```python
from build123d import *

# Parameters (mm, degrees)
SKETCH1_R                                       = 2.5
BOSS_EXTRUDE1_DEPTH                             = 35
CUT_EXTRUDE1_OUTLINE_W                          = 11.354248689
CUT_EXTRUDE1_OUTLINE_H                          = 14
CUT_EXTRUDE1_DEPTH                              = 10.980294351
CSK_FOR_M5_FLAT_HEAD_MACHINE_SCREW1_D           = 5.5
CSK_FOR_M5_FLAT_HEAD_MACHINE_SCREW1_DEPTH       = 13.347633298
CSK_FOR_M5_FLAT_HEAD_MACHINE_SCREW1_CSINK_D     = 10.4
CSK_FOR_M5_FLAT_HEAD_MACHINE_SCREW1_CSINK_ANGLE = 90
CSK_FOR_M5_FLAT_HEAD_MACHINE_SCREW1_TIP         = 1.652366702
SKETCH6_R                                       = 5.25
CUT_EXTRUDE2_DEPTH                              = 14
CUT_EXTRUDE3_START                              = -28
SKETCH6_2_R                                     = 5.25
CUT_EXTRUDE3_DEPTH                              = 14
CUT_EXTRUDE4_START                              = -56
SKETCH6_3_R                                     = 5.25
CUT_EXTRUDE4_DEPTH                              = 14


# Read off the part's stored shape, not the designer's step: Cut-Extrude1
with BuildPart() as part:
    # Sketch1 → Boss-Extrude1 (new, symmetric)
    with BuildSketch(Plane(origin=(0, 0, 0), x_dir=(1, 0, 0), z_dir=(0, 1, 0))):
        with BuildLine():
            Line((0, 0), (28, 0))
            Line((28, 0), (28, -1.5))
            ThreePointArc((28, -1.5), (34.920820135, -7.683011565), (25.645751311, -8))
            Line((25.645751311, -8), (2.645751311, -8))
            Line((2.645751311, -8), (0, -5))
            Line((0, -5), (0, 0))
        make_face()
        with Locations(Location((30.219676222, -5.980294351, 0), (0, 0, 270))):
            Circle(SKETCH1_R, mode=Mode.SUBTRACT)
    extrude(amount=BOSS_EXTRUDE1_DEPTH, both=True)

    # Cut-Extrude1 outline → Cut-Extrude1 (cut)
    with BuildSketch(Plane.XY):
        with Locations((31.322875655, 0)):
            Rectangle(CUT_EXTRUDE1_OUTLINE_W, CUT_EXTRUDE1_OUTLINE_H)
        with Locations((31.322875655, 28)):
            Rectangle(CUT_EXTRUDE1_OUTLINE_W, CUT_EXTRUDE1_OUTLINE_H)
        with Locations((31.322875655, -28)):
            Rectangle(CUT_EXTRUDE1_OUTLINE_W, CUT_EXTRUDE1_OUTLINE_H)
    extrude(amount=CUT_EXTRUDE1_DEPTH, mode=Mode.SUBTRACT)

    # CSK for M5 Flat Head Machine Screw1
    with Locations(Plane.XY.offset(8)):
        with Locations((12.432713767, 18), (12.432713767, -18)):
            CounterSinkHole(CSK_FOR_M5_FLAT_HEAD_MACHINE_SCREW1_D / 2, CSK_FOR_M5_FLAT_HEAD_MACHINE_SCREW1_CSINK_D / 2, depth=CSK_FOR_M5_FLAT_HEAD_MACHINE_SCREW1_DEPTH, counter_sink_angle=CSK_FOR_M5_FLAT_HEAD_MACHINE_SCREW1_CSINK_ANGLE)
            with Locations((0, 0, -(CSK_FOR_M5_FLAT_HEAD_MACHINE_SCREW1_DEPTH + CSK_FOR_M5_FLAT_HEAD_MACHINE_SCREW1_TIP / 2))):  # 118° drill point
                Cone(0, CSK_FOR_M5_FLAT_HEAD_MACHINE_SCREW1_D / 2, CSK_FOR_M5_FLAT_HEAD_MACHINE_SCREW1_TIP, mode=Mode.SUBTRACT)

    # Sketch6 → Cut-Extrude2 (cut)
    with BuildSketch(Plane(origin=(0, 35, 0), x_dir=(1, 0, 0), z_dir=(0, 1, 0))):
        with Locations((30.219676222, -5.980294351)):
            Circle(SKETCH6_R)
    extrude(amount=-CUT_EXTRUDE2_DEPTH, mode=Mode.SUBTRACT)

    # Sketch6<2> → Cut-Extrude3 (cut)
    with BuildSketch(Plane(origin=(0, 35, 0), x_dir=(1, 0, 0), z_dir=(0, 1, 0)).offset(CUT_EXTRUDE3_START)):
        with Locations((30.219676222, -5.980294351)):
            Circle(SKETCH6_2_R)
    extrude(amount=-CUT_EXTRUDE3_DEPTH, mode=Mode.SUBTRACT)

    # Sketch6<3> → Cut-Extrude4 (cut)
    with BuildSketch(Plane(origin=(0, 35, 0), x_dir=(1, 0, 0), z_dir=(0, 1, 0)).offset(CUT_EXTRUDE4_START)):
        with Locations((30.219676222, -5.980294351)):
            Circle(SKETCH6_3_R)
    extrude(amount=-CUT_EXTRUDE4_DEPTH, mode=Mode.SUBTRACT)


solid = part.part
```
The model under review builds one solid part; all positions refer to its coordinate system, in mm. A direction names the side the tool comes from. Round coordinates to 2 decimals unless told otherwise and drop trailing zeros. Order: outer loops, then holes, each group sorted by start corner. A loop starts at its lowest first (then second) coordinate and runs counter-clockwise, first axis right, second up.
Item 1: Add section A-A, the plane z = 10.25. State the section outline as (x, y) points, and give its area (3 significant figures).
Working result:
outline: (27.62, -21) - (32.82, -21) - (32.82, -7) - (27.62, -7) - close; (27.62, 7) - (32.82, 7) - (32.82, 21) - (27.62, 21) - close
area: 146 mm2
Item 2: Machinability: for faces 1 (the flat face through (1.34, 0.49, 6.52)), 2 (the flat face through (25.646, -28, 2)), 3 (the flat face through (25.646, 0, 2)), 4 (the flat face through (25.646, 28, 2)), 5 (the flat face through (13, 35, 4)), which of the approach directions +Z, -Z, +X, -X, +Y, -Y give a long, thin tool a straight path to every point of the face, cutting with its end or side? Answer none if there is none.
Working result:
face 1: +Z, -X, +Y, -Y
face 2: +Z, -Z, +X, -Y
face 3: +Z, -Z, +X
face 4: +Z, -Z, +X, +Y
face 5: +Z, -Z, +X, -X, +Y
Item 3: For pin 1 (1 mm diameter, centred on y = 0.5, z = 2, fed in from +X); pin 2 (5 mm diameter, centred on x = 30.5, z = 6.5, fed in from +Y); pin 3 (5 mm diameter, centred on x = 7, z = 9.5, fed in from -Y); pin 4 (6 mm diameter, centred on x = 12, y = 22.5, fed in from +Z), all flat-tipped, find the tip position at first contact; note any pin that passes through.
Working result:
pin 1: stops at x = 25.65
pin 2: stops at y = 21
pin 3: stops at y = -35
pin 4: stops at z = 8
Item 4: Add section C-C, the plane z = 2.75. State the section outline as (x, y) points.
Working result:
outline: (0, -35) - (25.65, -35) - (25.65, -21) - (34.04, -21) - (34.04, -7) - (25.65, -7) - (25.65, 7) - (34.04, 7) - (34.04, 21) - (25.65, 21) - (25.65, 35) - (0, 35) - close; hole circle Ø5.5 at (12.43, -18); hole circle Ø5.5 at (12.43, 18)
Item 5: Draft analysis for pull direction Z (two halves, no side actions). For faces 6 (the cylindrical face through (24.98, 28.1, 5.64)), 7 (the cylindrical face through (32.698, -14.098, 5.655)), 8 (the flat face through (14, 0, 0)), 9 (the cylindrical face through (9.8, -17.2, 2.7)), state which applies: released by +Z, released by -Z, zero draft, split by the parting line, or undercut.
Working result:
face 6: undercut
face 7: undercut
face 8: released by -Z
face 9: zero draft
Item 6: To check wall thickness, follow probe 1 along Y at (x, z) = (13, 1); probe 2 along Y at (x, z) = (13, 7.75); probe 3 along X at (y, z) = (-18, 4.45). State the ranges of each line that lie inside material, in increasing order.
Working result:
probe 1: y = -35 to -20.69, -15.31 to 15.31, 20.69 to 35
probe 2: y = -35 to -22.92, -13.08 to 13.08, 22.92 to 35
probe 3: x = 0 to 9.68, 15.18 to 28.24, 32.2 to 34.98
Item 7: Add section B-B, the plane y = 18. State the section outline as (x, z) points.
Working result:
outline: (0, 0) - (9.68, 0) - (9.68, 5.55) - (7.23, 8) - (2.65, 8) - (0, 5) - close; (15.18, 0) - (28, 0) - (28, 1.5) arc R5 ccw (long way) to (25.65, 8) - (17.63, 8) - (15.18, 5.55) - close; hole circle Ø5 at (30.22, 5.98)
Item 8: Add section D-D, the plane x = 23. State the section outline as (y, z) points, and give its area (3 significant figures).
Working result:
outline: (-35, 0) - (35, 0) - (35, 8) - (-35, 8) - close
area: 560 mm2
